Design review of the part built by this model. Coordinates are the model's own, in mm. A direction names the side the tool comes from. Coordinates: 2 decimals unless noted, no trailing zeros. Loops run counter-clockwise (first coordinate to the right, second up) from the corner with the lowest first, then second, coordinate; pieces in that order, holes last. Notation, with made-up numbers: (60.5, 18) - (69.5, 18) arc R13 cw to (69.5, 26) - close; hole circle Ø4 at (40, 69.25). An arc over 180 degrees is marked (long way). Answer in a Markdown table with one row per item. Add a question column.
(1) The part is to be moulded in two halves that separate along X. For faces 4 (the face through (47.5, 0, 13)), 5 (the face through (-47.5, 0, 13)), 6 (the face through (-1, 17.5, 13)), 7 (the face through (-39.7, -0.2, 16.5)), say which applies: released by +X, released by -X, zero draft, split by the parting line, or undercut.
(2) We need section D-D, the plane x = -10.5. Write out the cut boundary in (y, z), plus the area to 3 significant figures.
(3) We need section B-B, the plane y = 0. Write out the cut boundary in (x, z).
(4) For faces 1 (the face through (37.834, -13.769, 8.112)), 2 (the face through (-23.778, -13.066, 20.916)), 3 (the face through (46, 0, 19)), list the 3-axis set-ups (+Z, -Z, +X, -X, +Y, -Y) from which the entire face can be reached by the end or side of a thin tool; tool diameter is ignored.
(5) To check wall thickness, follow L1, parallel to X at y = 13.5, z = 4; L2, parallel to X at y = -13.5, z = 11.75; L3, parallel to X at y = 13.5, z = 18.25. State the ranges of each line that lie inside material, in increasing order. Write a range as [from, to].
(6) Clearance check with flat-ended pins moving along their axes: pin 1 (2 mm diameter, centred on x = -26.5, y = 13.5, fed in from +Z); pin 2 (10 mm diameter, centred on x = -13.5, y = 6.5, fed in from +Z); pin 3 (6 mm diameter, centred on x = -11, y = 4.5, fed in from +Z). State where each tip first meets the part, or that it passes through.
(7) We need section A-A, the plane y = -13.5. Give the number of separate pieces and of enclosed holes in the cut face, plus the area to 3 significant figures.
Solid Edge part; units mm, degrees
sketch "Sketch1" plane through (0, 0, 0) normal (0, 0, 1) x (1, 0, 0)
  line L0 (47.5, -17.5) -> (-47.5, -17.5)
  line L1 (-47.5, -17.5) -> (-47.5, 17.5)
  line L2 (-47.5, 17.5) -> (47.5, 17.5)
  line L3 (47.5, 17.5) -> (47.5, -17.5)
  dimension "D1" = 47.5
  dimension "D2" = 47.5
extrude "Protrusion1" add sketch "Sketch1" along normal blind 27
sketch "Sketch2" plane through (0, 0, 27) normal (0, 0, 1) x (1, 0, 0)
  line L0 (3.77, 15) -> (3.77, 17)
  line L1 (3.77, 17) -> (30.77, 17)
  line L2 (30.77, 17) -> (30.77, 8)
  line L3 (36.5, 8) -> (30.77, 8)
  line L4 (36.5, 9.25) -> (36.5, 8)
  line L5 (37.5, 9.25) -> (36.5, 9.25)
  line L6 (37.5, 10.5) -> (37.5, 9.25)
  line L7 (42.5, 10.5) -> (37.5, 10.5)
  line L8 (42.5, 9.25) -> (42.5, 10.5)
  line L9 (42.5, 9.25) -> (43.5, 9.25)
  line L10 (43.5, 9.25) -> (43.5, 8)
  line L11 (43.5, 8) -> (47.5, 8)
  line L12 (47.5, 8) -> (47.5, 0)
  line L13 (-47.5, 0) -> (-47.5, 8)
  line L14 (-43.23, 8) -> (-47.5, 8)
  line L15 (-43.23, 8) -> (-43.23, 9.25)
  line L16 (-43.23, 9.25) -> (-42.23, 9.25)
  line L17 (-42.23, 9.25) -> (-42.23, 10.5)
  line L18 (-42.23, 10.5) -> (-37.23, 10.5)
  line L19 (-37.23, 10.5) -> (-37.23, 9.25)
  line L20 (-37.23, 9.25) -> (-36.23, 9.25)
  line L21 (-36.23, 9.25) -> (-36.23, 8)
  line L22 (-21.23, 8) -> (-36.23, 8)
  line L23 (-21.23, 8) -> (-21.23, 15)
  line L24 (-21.23, 15) -> (3.77, 15)
  dimension "D1" = 3.77
revolve "RevolvedCutout1" cut sketch "Sketch2" angle 360 about axis through (47.5, 0, 27) along (-1, 0, 0)
sketch "Sketch3" plane through (0, -17.5, 13.5) normal (0, -1, 0) x (1, 0, 0)
  line L0 (3.77, 5) -> (30.77, 5)
  line L1 (30.77, 5) -> (30.77, 13.5)
  line L2 (30.77, 13.5) -> (3.77, 13.5)
  line L3 (3.77, 13.5) -> (3.77, 5)
extrude "Extrusionsausschnitt_1" cut sketch "Sketch3" against normal blind 7.5
sketch "Sketch4" plane through (17.27, -16.1112, 18.5) normal (0, 0, 1) x (1, 0, 0)
  line L0 (-13.5, 6.1112) -> (13.5, 6.1112)
  line L1 (-13.5, -1.3888) -> (-13.5, 6.1112)
  line L2 (13.5, -1.3888) -> (-13.5, -1.3888)
  line L3 (14.996, -1.3888) -> (13.5, -1.3888)
  line L4 (14.996, 6.1112) -> (14.996, -1.3888)
  line L5 (13.5, 6.1112) -> (14.996, 6.1112)
  dimension "D1" = 13.5
  dimension "D2" = 13.5
extrude "Extrusionsausschnitt_2" cut sketch "Sketch4" along normal mid plane 100
hole "Bohrung_1" at (-25.73, 13.5, 27) direction (0, 0, -1) diameter 4 depth 12
hole "Hole1" at (39.883, -13.5, 27) direction (0, 0, -1) diameter 4 depth 12
hole "Hole2" at (-25.73, -13.5, 27) direction (0, 0, -1) diameter 4 depth 12
hole "Hole3" at (-43, -13.5, 27) direction (0, 0, -1) diameter 4 depth 12
hole "Hole4" at (-43, 13.5, 27) direction (0, 0, -1) diameter 4 depth 12
hole "Hole5" at (44, 13.5, 27) direction (0, 0, -1) diameter 4 depth 12
hole "Bohrung_8" at (-33.23, -13.5, 0) direction (0, 0, 1) diameter 4.134 depth 16
hole "Hole6" at (39.88, 13.5, 0) direction (0, 0, 1) diameter 4.134 depth 16
hole "Hole7" at (39.883, -13.5, 0) direction (0, 0, 1) diameter 4.134 depth 16
hole "Hole8" at (-33.23, 13.5, 0) direction (0, 0, 1) diameter 4.134 depth 16
properties material "Aluminium, 1060"
Responses:
| question | item | result |
|---|---|---|
| 1 | face 4 | released by +X |
| 1 | face 5 | released by -X |
| 1 | face 6 | zero draft |
| 1 | face 7 | undercut |
| 2 | outline | (-17.5, 0) - (17.5, 0) - (17.5, 27) - (15, 27) arc R15 cw to (-15, 27) - (-17.5, 27) - close |
| 2 | area | 592 mm2 |
| 3 | outline | (-47.5, 0) - (47.5, 0) - (47.5, 19) - (43.5, 19) - (43.5, 17.75) - (42.5, 17.75) - (42.5, 16.5) - (37.5, 16.5) - (37.5, 17.75) - (36.5, 17.75) - (36.5, 19) - (30.77, 19) - (30.77, 10) - (3.77, 10) - (3.77, 12) - (-21.23, 12) - (-21.23, 19) - (-36.23, 19) - (-36.23, 17.75) - (-37.23, 17.75) - (-37.23, 16.5) - (-42.23, 16.5) - (-42.23, 17.75) - (-43.23, 17.75) - (-43.23, 19) - (-47.5, 19) - close |
| 4 | face 1 | -Z |
| 4 | face 2 | +Z |
| 4 | face 3 | +Z, +X, -X |
| 5 | L1 | x = [-47.5, -35.3], [-31.16, 37.81], [41.95, 47.5] |
| 5 | L2 | x = [-47.5, -35.3], [-31.16, 3.77], [32.27, 37.82], [41.95, 47.5] |
| 5 | L3 | x = [-47.5, -45], [-41, -27.73], [-23.73, 3.77], [30.77, 42], [46, 47.5] |
| 6 | pin 1 | stops at z = 15 |
| 6 | pin 2 | stops at z = 17.37 |
| 6 | pin 3 | stops at z = 14.01 |
| 7 | separate pieces | 3 |
| 7 | enclosed holes | 0 |
| 7 | area | 1,360 mm2 |
